```python
from build123d import *

# Parameters (mm, degrees)
BOSS_EXTRUDE1_DEPTH = 3
SKETCH2_W           = 19
SKETCH2_H           = 24.344098819
BOSS_EXTRUDE2_DEPTH = 5


with BuildPart() as part:
    # Sketch1 → Boss-Extrude1 (new body)
    with BuildSketch(Plane.XY):
        with BuildLine():
            Line((11.419301697, 73.454544617), (11.419301697, -43.242123234))
            ThreePointArc((11.419301697, -43.242123234), (-62.561825873, 15.106210692), (11.419301697, 73.454544617))
        make_face()
    extrude(amount=BOSS_EXTRUDE1_DEPTH)

    # Sketch2 → Boss-Extrude2 (add)
    with BuildSketch(Plane.XY.offset(3)):
        with Locations((-18.580698303, -37.949042382)):
            Rectangle(SKETCH2_W, SKETCH2_H)
    extrude(amount=-BOSS_EXTRUDE2_DEPTH)


solid = part.part
```
For this review, take the finished solid that the model builds, in its own axes (mm). A direction names the side the tool comes from. Round coordinates to 2 decimals unless told otherwise and drop trailing zeros. Order: outer loops, then holes, each group sorted by start corner. A loop starts at its lowest first (then second) coordinate and runs counter-clockwise, first axis right, second up.
Q1. Wall thickness on line 1 (X direction, y = -42, z = -0.6); line 2 (Y direction, x = -23.5, z = -0.2); line 3 (Z direction, x = -18.5, y = 40): over which ranges is each line inside the solid? List them lowest first.
Findings below:
line 1: x = -28.08 to -9.08
line 2: y = -50.12 to -25.78
line 3: z = 0 to 3
Q2. We need section A-A, the plane x = -12. Give the boundary of the cut face in (y, z), plus the area to 3 significant figures.
Findings below:
outline: (-50.12, -2) - (-25.78, -2) - (-25.78, 0) - (74.36, 0) - (74.36, 3) - (-50.12, 3) - close
area: 422 mm2
Q3. Insertion check: P1, Ø3, axis at y = 32.5, z = -0.5, coming from the -X side; P2, Ø1.5, axis at y = -36.5, z = -0.5, coming from the +X side. Each pin has a flat end and moves straight along its axis. Give the tip position at first contact, or say it passes through.
Findings below:
P1: stops at x = -60.39
P2: stops at x = 11.42
Q4. Machinability: for faces 1 (the flat face through (-28.081, -41, 0)), 2 (the cylindrical face through (1.369, -44.765, 1.479)), which of the approach directions +Z, -Z, +X, -X, +Y, -Y give a long, thin tool a straight path to every point of the face, cutting with its end or side? Answer none if there is none.
Findings below:
face 1: -Z, -X, -Y
face 2: +Z, -Z, -Y
Q5. We need section C-C, the plane y = 23. Give the boundary of the cut face in (x, z).
Findings below:
outline: (-62.04, 0) - (11.42, 0) - (11.42, 3) - (-62.04, 3) - close
Q6. We need section B-B, the plane z = 1.75. Give the boundary of the cut face in (x, y).
Findings below:
outline: (-28.08, -50.12) - (-9.08, -50.12) - (-9.08, -44.54) arc R60 ccw to (11.42, -43.24) - (11.42, 73.45) arc R60 ccw to (-28.08, -39.2) - close
Q7. We need section D-D, the plane x = -48.5. Give the boundary of the cut face in (y, z).
Findings below:
outline: (-23.49, 0) - (53.7, 0) - (53.7, 3) - (-23.49, 3) - close
